Autodesk Inventor part; units mm, degrees
ref_plane "YZ Plane" through (0, 0, 0) normal (1, 0, 0) x (0, 1, 0)
ref_plane "XZ Plane" through (0, 0, 0) normal (0, 1, 0) x (-1, 0, 0)
ref_plane "XY Plane" through (0, 0, 0) normal (0, 0, 1) x (1, 0, 0)
sketch "Sketch7" plane through (0, 0, 0) normal (0, 1, 0) x (-1, 0, 0)
  circle A0 centre (-43.3, 100) radius 13.3 construction
  circle A1 centre (-43.3, 100) radius 31.3 construction
  line L0 (-86.6, 0) -> (0, 0)
  line L1 (0, 0) -> (0, 200)
  line L2 (0, 200) -> (-86.6, 200)
  line L3 (-86.6, 200) -> (-86.6, 0)
  line L4 (0, 200) -> (-86.6, 200)
  line L5 (-46.3, 68.8441) -> (-46.3, 87.0428)
  line L6 (-40.3, 68.8441) -> (-40.3, 87.0428)
  arc A2 (-46.3, 87.0428) -> (-40.3, 87.0428) centre (-43.3, 100) ccw
  arc A3 (-46.3, 68.8441) -> (-40.3, 68.8441) centre (-43.3, 100) ccw
  line L7 (-19.1481, 80.0908) -> (-32.0165, 92.9592)
  arc A4 (-23.3908, 75.8481) -> (-19.1481, 80.0908) centre (-43.3, 100) ccw
  line L8 (-23.3908, 75.8481) -> (-36.2592, 88.7165)
  arc A5 (-36.2592, 88.7165) -> (-32.0165, 92.9592) centre (-43.3, 100) ccw
  line L9 (-12.1441, 103) -> (-30.3428, 103)
  arc A6 (-12.1441, 97) -> (-12.1441, 103) centre (-43.3, 100) ccw
  line L10 (-12.1441, 97) -> (-30.3428, 97)
  arc A7 (-30.3428, 97) -> (-30.3428, 103) centre (-43.3, 100) ccw
  line L11 (-23.3908, 124.1519) -> (-36.2592, 111.2835)
  arc A8 (-19.1481, 119.9092) -> (-23.3908, 124.1519) centre (-43.3, 100) ccw
  line L12 (-19.1481, 119.9092) -> (-32.0165, 107.0408)
  arc A9 (-32.0165, 107.0408) -> (-36.2592, 111.2835) centre (-43.3, 100) ccw
  line L13 (-46.3, 131.1559) -> (-46.3, 112.9572)
  arc A10 (-40.3, 131.1559) -> (-46.3, 131.1559) centre (-43.3, 100) ccw
  line L14 (-40.3, 131.1559) -> (-40.3, 112.9572)
  arc A11 (-40.3, 112.9572) -> (-46.3, 112.9572) centre (-43.3, 100) ccw
  line L15 (-67.4519, 119.9092) -> (-54.5835, 107.0408)
  arc A12 (-63.2092, 124.1519) -> (-67.4519, 119.9092) centre (-43.3, 100) ccw
  line L16 (-63.2092, 124.1519) -> (-50.3408, 111.2835)
  arc A13 (-50.3408, 111.2835) -> (-54.5835, 107.0408) centre (-43.3, 100) ccw
  line L17 (-74.4559, 97) -> (-56.2572, 97)
  arc A14 (-74.4559, 103) -> (-74.4559, 97) centre (-43.3, 100) ccw
  line L18 (-74.4559, 103) -> (-56.2572, 103)
  arc A15 (-56.2572, 103) -> (-56.2572, 97) centre (-43.3, 100) ccw
  line L19 (-63.2092, 75.8481) -> (-50.3408, 88.7165)
  arc A16 (-67.4519, 80.0908) -> (-63.2092, 75.8481) centre (-43.3, 100) ccw
  line L20 (-67.4519, 80.0908) -> (-54.5835, 92.9592)
  arc A17 (-54.5835, 92.9592) -> (-50.3408, 88.7165) centre (-43.3, 100) ccw
  line L21 (-86.6, 200) -> (-86.6, 0)
  point P0 (-43.3, 200)
  point P1 (-86.6, 100)
  point P2 (-43.3, 200)
  point P3 (-43.3, 86.7)
  point P4 (-33.8955, 90.5955)
  point P5 (-30, 100)
  point P6 (-33.8955, 109.4045)
  point P7 (-43.3, 113.3)
  point P8 (-52.7045, 109.4045)
  point P9 (-56.6, 100)
  point P10 (-52.7045, 90.5955)
  dimension "d36" = 18
  dimension "d37" = 6
  dimension "d38" = 360
  dimension "d39" = 30
  dimension "d42" = 100
  dimension "d43" = 200
  dimension "d44" = 86.6
extrude "Extrusion3" add sketch "Sketch7" along normal blind 3.3
sketch "Sketch8" plane through (0, 3.3, 0) normal (0, 1, 0) x (1, 0, 0)
  line L0 (7.3, -150.05) -> (79.3, -150.05)
  line L1 (79.3, -150.05) -> (79.3, -49.95)
  line L2 (79.3, -49.95) -> (7.3, -49.95)
  line L3 (7.3, -49.95) -> (7.3, -150.05)
  line L4 (4.1, -153.25) -> (82.5, -153.25)
  line L5 (82.5, -153.25) -> (82.5, -46.75)
  line L6 (82.5, -46.75) -> (4.1, -46.75)
  line L7 (4.1, -46.75) -> (4.1, -153.25)
  line L8 (86.6, 0) -> (0, 0)
  line L9 (0, 0) -> (0, -200)
  dimension "d47" = 3.2
  dimension "d48" = 3.2
  dimension "d49" = 3.2
  dimension "d50" = 3.2
  dimension "largo_bateria" = 100.1
  dimension "ancho_bateria" = 72
  dimension "d54" = 7.3
  dimension "d55" = 49.95
extrude "Extrusion4" cut sketch "Sketch8" against normal blind 1
equation "\"d36\" = 1.5 * d41"
equation "\"d37\" = 0.2 * d39"
equation "\"d42\" = 0.5 * largo_base"
equation "\"d43\" = largo_base"
equation "\"d48\" = d47"
equation "\"d49\" = d47"
equation "\"d50\" = d47"
equation "\"d55\" = 0.5 * largo_base - 0.5 * largo_bateria"
equation "\"espesor\" = 3.2"
properties part number "cuerpo-base-bateria"
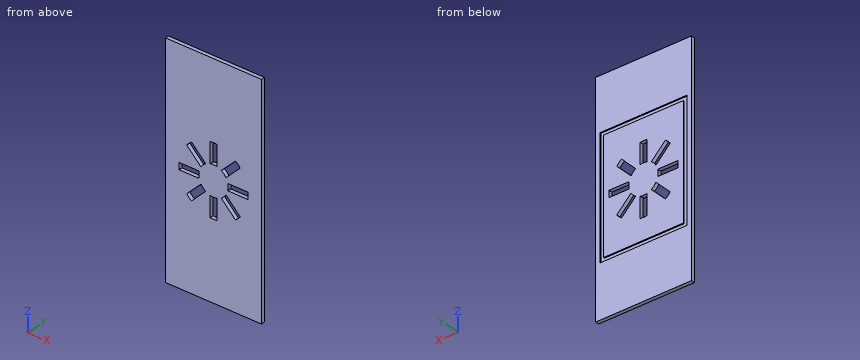
Here's how the part is built. I have some questions about the finished solid (model axes, mm). Round coordinates to 2 decimals unless told otherwise and drop trailing zeros. Write each loop counter-clockwise with the first axis right and the second up, starting at its lowest first coordinate (ties: lowest second). Pieces come first, ordered by that corner, then holes. Notation, with made-up numbers: (57, -35.75) -> (68, -35.75) arc R8 cw to (68, -31.75) -> close; hole circle Ø5 at (25.25, -28.75). An arc over 180 degrees is marked (long way). One line per item, written item: value.
1) Suppose I cut it at C-C on z = 115.5. List the corners of the cut face in (x, y) for me.
Filled sheet:
outline: (0, 0) -> (23.56, 0) -> (23.56, 3.3) -> (7.3, 3.3) -> (7.3, 2.3) -> (4.1, 2.3) -> (4.1, 3.3) -> (0, 3.3) -> close; (32.04, 0) -> (40.3, 0) -> (40.3, 3.3) -> (32.04, 3.3) -> close; (46.3, 0) -> (54.56, 0) -> (54.56, 3.3) -> (46.3, 3.3) -> close; (63.04, 0) -> (86.6, 0) -> (86.6, 3.3) -> (82.5, 3.3) -> (82.5, 2.3) -> (79.3, 2.3) -> (79.3, 3.3) -> (63.04, 3.3) -> close
2) Suppose I cut it at D-D on z = 63.5. List the corners of the cut face in (x, y) for me, plus the area to 3 significant figures.
Filled sheet:
outline: (0, 0) -> (86.6, 0) -> (86.6, 3.3) -> (82.5, 3.3) -> (82.5, 2.3) -> (79.3, 2.3) -> (79.3, 3.3) -> (7.3, 3.3) -> (7.3, 2.3) -> (4.1, 2.3) -> (4.1, 3.3) -> (0, 3.3) -> close
area: 279 mm2
3) Suppose I cut it at A-A on x = 70. List the corners of the cut face in (y, z) for me, plus the area to 3 significant figures.
Filled sheet:
outline: (0, 0) -> (3.3, 0) -> (3.3, 46.75) -> (2.3, 46.75) -> (2.3, 49.95) -> (3.3, 49.95) -> (3.3, 97) -> (0, 97) -> close; (0, 103) -> (3.3, 103) -> (3.3, 150.05) -> (2.3, 150.05) -> (2.3, 153.25) -> (3.3, 153.25) -> (3.3, 200) -> (0, 200) -> close
area: 634 mm2
4) Suppose I cut it at B-B on x = 60.5. List the corners of the cut face in (y, z) for me.
Filled sheet:
outline: (0, 0) -> (3.3, 0) -> (3.3, 46.75) -> (2.3, 46.75) -> (2.3, 49.95) -> (3.3, 49.95) -> (3.3, 78.56) -> (0, 78.56) -> close; (0, 87.04) -> (3.3, 87.04) -> (3.3, 97) -> (0, 97) -> close; (0, 103) -> (3.3, 103) -> (3.3, 112.96) -> (0, 112.96) -> close; (0, 121.44) -> (3.3, 121.44) -> (3.3, 150.05) -> (2.3, 150.05) -> (2.3, 153.25) -> (3.3, 153.25) -> (3.3, 200) -> (0, 200) -> close
5) If I drill on line 1 (X direction, y = 1.8, z = 99.5); line 2 (Z direction, x = 8, y = 2.75); line 3 (Z direction, x = 44, y = 2.2), over which ranges is the centre line in solid material (lowest first)? Write a range as [from, to].
Filled sheet:
line 1: x = [0, 12], [30.01, 56.59], [74.6, 86.6]
line 2: z = [0, 46.75], [49.95, 150.05], [153.25, 200]
line 3: z = [0, 68.71], [86.72, 113.28], [131.29, 200]
